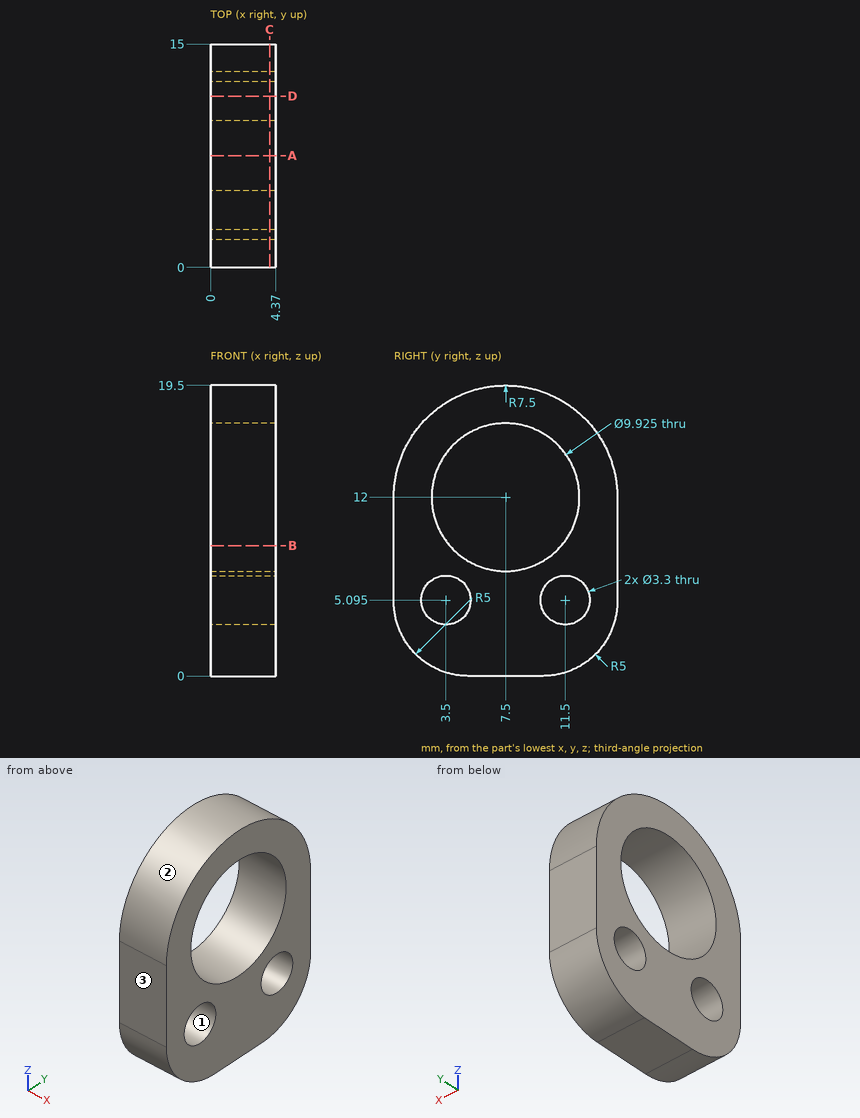
The figure shows three views and two pictorial views of one solid part (mm, origin at its lowest corner). Answer the questions. Coordinates: 2 decimals unless noted, no trailing zeros. Write each loop counter-clockwise with the first axis right and the second up, starting at its lowest first coordinate (ties: lowest second). Pieces come first, ordered by that corner, then holes. Notation, with made-up numbers: (-7.75, -25.5) -> (13.25, -25.5) arc R9 cw to (13.25, -12.5) -> close; hole circle Ø5 at (75, 7). An arc over 180 degrees is marked (long way). Return JSON: item names as keys, results as strings.
(1) For a pull along Y with two mould halves and no side action, classify the marked faces 1, 2 and 3 as pulls with the +Y half, pulls with the -Y half, needs draft (parallel to the pull), parting line crosses it, or undercut.
Answers below:
{"face 1": "undercut", "face 2": "parting line crosses it", "face 3": "pulls with the -Y half"}
(2) The part is cut by section C-C on x = 3.95. State how many separate pieces and enclosed holes the cut face has, then the cut area to 3 significant figures.
Answers below:
{"separate pieces": "1", "enclosed holes": "3", "area": "163 mm^2"}
(3) The part is cut by section B-B on z = 8.75. Give the vertices of the cut face in (x, y), then the cut area to 3 significant figures.
Answers below:
{"outline": "(0, 0) -> (4.37, 0) -> (4.37, 3.75) -> (0, 3.75) -> close; (0, 11.25) -> (4.37, 11.25) -> (4.37, 15) -> (0, 15) -> close", "area": "32.8 mm^2"}
(4) The part is cut by section D-D on y = 11.5. Give the vertices of the cut face in (x, z) (1 decimal).
Answers below:
{"outline": "(0, 0.2) -> (4.4, 0.2) -> (4.4, 3.4) -> (0, 3.4) -> close; (0, 6.7) -> (4.4, 6.7) -> (4.4, 9.1) -> (0, 9.1) -> close; (0, 14.9) -> (4.4, 14.9) -> (4.4, 18.3) -> (0, 18.3) -> close"}
(5) Consider line 1 along Y through (x, z) = (1.95, 4); line 2 along Z through (x, y) = (0.75, 8.25); line 3 along Y through (x, z) = (3.9, 4.25). Determine where each line is inside the solid, lowest interval first. Write a range as from..to.
Answers below:
{"line 1": "0.1..2.27, 4.73..10.27, 12.73..14.9", "line 2": "0..7.09, 16.91..19.46", "line 3": "0.06..2.08, 4.92..10.08, 12.92..14.94"}
(6) The part is cut by section A-A on y = 7.5. Give the vertices of the cut face in (x, z).
Answers below:
{"outline": "(0, 0) -> (4.37, 0) -> (4.37, 7.04) -> (0, 7.04) -> close; (0, 16.96) -> (4.37, 16.96) -> (4.37, 19.5) -> (0, 19.5) -> close"}
